Can you work these out from the drawing? Everything is in mm from the part's minimum corner. A direction names the side the tool comes from. Round coordinates to 2 decimals unless told otherwise and drop trailing zeros. Order: outer loops, then holes, each group sorted by start corner. A loop starts at its lowest first (then second) coordinate and runs counter-clockwise, first axis right, second up. Notation, with made-up numbers: M -5.75,52.25 L 23.25,52.25 A24 cw 23.25,85.25 Z; hole C 72.25,78 d1. An arc over 180 degrees is marked long. Write each question's results on one line, items separated by ' | '. Start each with the question number.
1. For the marked faces 1 and 2, which set-ups out of +Z, -Z, +X, -X, +Y, -Y let a thin tool reach every point of the face, with its end or its side?
2. Suppose I cut it at B-B on x = 4.95. Write out the boundary of the cut face in (y, z) (1 decimal), and give its area (3 significant figures).
3. We'd pull the mould along X, two halves only. Please class the marked faces 3, 4 and 5: released by +X, released by -X, zero draft, split by the parting line, or undercut.
4. Suppose I cut it at C-C on z = 2. Write out the boundary of the cut face in (x, y), and give its area (3 significant figures).
5. I'm going to push flat-ended pins straight in: pin 1 (1 mm diameter, centred on x = 4, z = 5.5, fed in from +Y) (1 decimal); pin 2 (1.8 mm diameter, centred on y = 3, z = 1, fed in from +X); pin 3 (2 mm diameter, centred on x = 3, z = 11, fed in from -Y); pin 4 (3 mm diameter, centred on x = 4.5, z = 10, fed in from +Y). Where does each tip first touch, or does it pass through?
6. Please list where these lines run through material, in increasing order: L1, parallel to Z at x = 3.1, y = 3.15 (1 decimal); L2, parallel to Z at x = 2.1, y = 1 (1 decimal); L3, parallel to Y at x = 1.9, z = 1.5 (1 decimal).
7. Suppose I cut it at A-A on z = 12.5. Write out the boundary of the cut face in (x, y) (1 decimal).
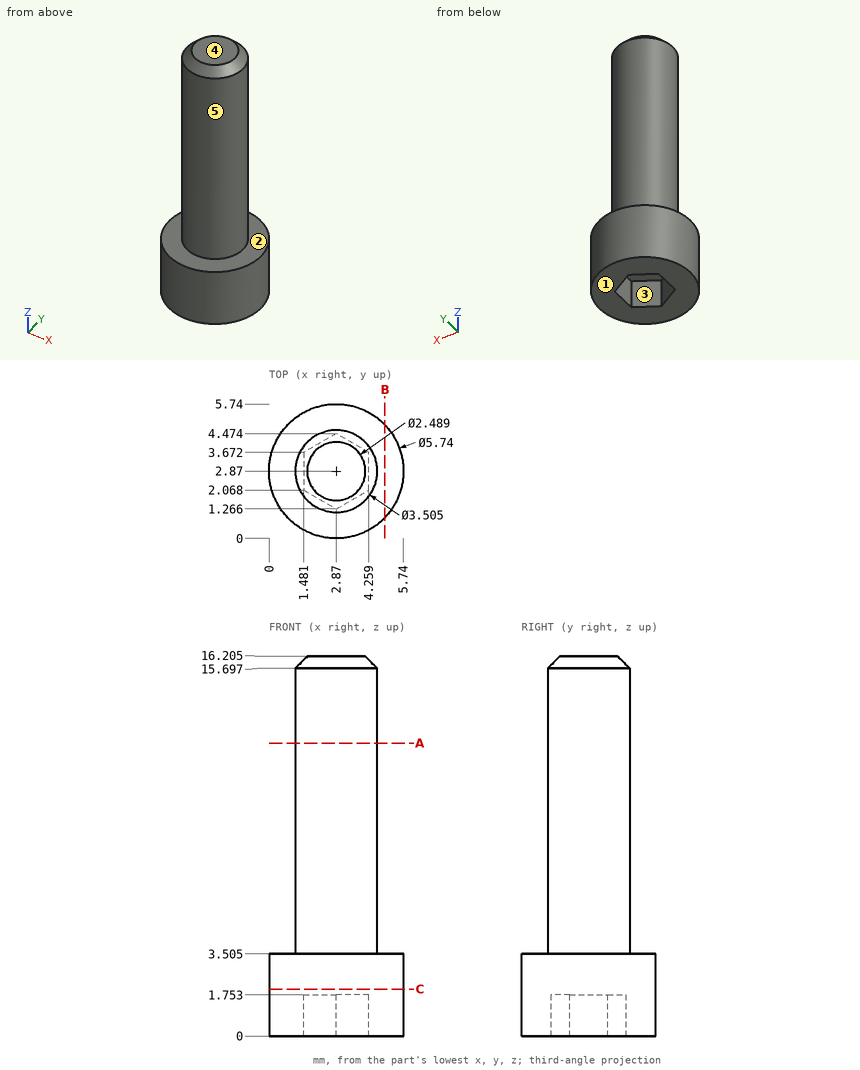
Filled sheet:
1) face 1: -Z, +X, -X, +Y, -Y | face 2: +Z
2) outline: M 0.9,0 L 4.8,0 L 4.8,3.5 L 0.9,3.5 Z | area: 13.9 mm^2
3) face 3: undercut | face 4: zero draft | face 5: split by the parting line
4) outline: C 2.87,2.87 d5.74 | area: 25.9 mm^2
5) pin 1: stops at y = 4.5 | pin 2: stops at x = 5.74 | pin 3: stops at y = 1.12 | pin 4: stops at y = 4.62
6) L1: z = 1.8 to 16.2 | L2: z = 0 to 3.5 | L3: y = 0.2 to 1.8, 3.9 to 5.6
7) outline: C 2.9,2.9 d3.5
